Geometry: final body of the model. Coordinates: model frame, mm. A direction names the side the tool comes from. Round coordinates to 2 decimals unless told otherwise and drop trailing zeros. Order: outer loops, then holes, each group sorted by start corner. A loop starts at its lowest first (then second) coordinate and runs counter-clockwise, first axis right, second up. Notation, with made-up numbers: (85.5, 35.5) - (103.5, 35.5) arc R14 cw to (103.5, 61.5) - close; hole circle Ø6 at (30.25, 59). An arc over 180 degrees is marked (long way). Put each result on its own line as item: value. Start each with the question number.
(1) Section C-C (z = -8). Output: boundary loops of the cut face in (x, y).
(2) Pin query (flat end, axial travel): P1, Ø2, axis at x = 30.5, y = -4.5, coming from the -Z side; P2, Ø2, axis at x = -6.5, y = 57.5, coming from the -Z side; P3, Ø6, axis at x = 26.5, z = -12, coming from the -Y side. Return the tip coordinate at first contact, or that it passes through.
(3) Material intervals for L1, parallel to Y at x = -6.5, z = -17.75; L2, parallel to Y at x = -6.5, z = -13.75; L3, parallel to Y at x = 29.5, z = -10, sorted ascending. Write a range as [from, to].
(4) Access query for faces 4 (the face through (0.15, -11.25, 1.73)), 5 (the face through (0, 61, -16)), 6 (the face through (0, 55, -16)). Directions: +Z, -Z, +X, -X, +Y, -Y. A direction counts if a zero-diameter tool reaches every point of the face in a straight line with its end or side. Return the directions, or none.
(5) Section A-A (x = 0). Output: boundary loops of the cut face in (y, z).
(6) Pull-direction query (Z, two-part tool) for faces 1 (the face through (-0.15, 11.25, 1.73)), 2 (the face through (0, -55, -16)), 3 (the face through (10.892, 34.587, 1.745)); classes: released by +Z, released by -Z, zero draft, split by the parting line, or undercut.
(7) Section B-B (y = 0). Output: boundary loops of the cut face in (x, z), and give its area (3 significant figures).
Autodesk Inventor part; units mm, degrees
ref_plane "Work Plane2" through (0, 61, 0) normal (0, 1, 0) x (-1, 0, 0)
ref_plane "YZ Plane" through (0, 0, 0) normal (1, 0, 0) x (0, 1, 0)
ref_plane "XY Plane" through (0, 0, 0) normal (0, 0, 1) x (1, 0, 0)
sketch "Sketch1" plane through (0, 0, 0) normal (0, 0, 1) x (1, 0, 0)
  circle A0 centre (0, 0) radius 11.25
  line L0 (-9, 6.75) -> (-9, -6.75)
  line L1 (9, 6.75) -> (9, -6.75)
  circle A1 centre (0, 0) radius 32.5
  dimension "d0" = 22.5
  dimension "d1" = 18
  dimension "d2" = 65
extrude "Extrusion1" add sketch "Sketch1" along normal blind 3.5 contours A0 L1 | L0 A0 | A1
sketch "Sketch2" plane through (0, 0, 0) normal (1, 0, 0) x (0, 1, 0)
  line L0 (32.5, 0) -> (-32.5, 0)
  line L1 (32.5, 0) -> (55.5, -21.5)
  line L2 (55.5, -21.5) -> (62.5, -21.5)
  line L3 (62.5, -21.5) -> (62.5, -10.5)
  line L4 (32.5, 3.5) -> (-32.5, 3.5)
  line L5 (32.5, 3.5) -> (62.5, -10.5)
  line L6 (0, 0) -> (0, -19.375) construction
  line L7 (32.5, 3.5) -> (32.5, 0)
  dimension "d8" = 7
  dimension "d9" = 25
  dimension "d10" = 11
  dimension "d11" = 30
revolve "Revolution1" add sketch "Sketch2" angle 360 about axis through (0, 0, 0) along (0, 0, -1)
fillet "Fillet1" radius 10 1 edges at (0, -32.5, 3.5)
ref_plane "Work Plane2" through (0, 61, 0) normal (0, 1, 0) x (-1, 0, 0)
sketch "Sketch3" plane through (0, 61, 0) normal (0, 1, 0) x (-1, 0, 0)
  circle A0 centre (0, -16) radius 4.5
  line L0 (4.5, -16) -> (4.5, -20.5)
  line L1 (-4.5, -20.5) -> (-4.5, -16)
  line L2 (-62.5, -21.5) -> (62.5, -21.5)
  line L3 (62.5, -21.5) -> (62.5, -11.7) construction
  line L4 (62.5, -10.5) -> (62.5, -21.5)
  line L5 (-9, 0) -> (9, 0)
  line L6 (-4.5, -20.5) -> (4.5, -20.5)
  point P0 (0, 0)
  point P1 (0, 0)
  point P2 (0, -20.5)
  dimension "d14" = 9
  dimension "d22" = 1
extrude "Extrusion2" cut sketch "Sketch3" against normal blind 6
sketch "Sketch4" plane through (0, 0, 3.5) normal (0, 0, 1) x (1, 0, 0)
  circle A0 centre (0, 45) radius 9
  point P0 (0, 0)
  dimension "d25" = 45
  dimension "d26" = 18
extrude "Extrusion3" [suppressed]
pattern_circular "Circular Pattern1" [suppressed]
mirror "Mirror1" about plane through (0, 0, 0) normal (0, 1, 0) of "Extrusion2"
sketch "Sketch5" plane through (0, 0, -21.5) normal (0, 0, -1) x (-1, 0, 0)
  circle A0 centre (0, 0) radius 62.5
  circle A1 centre (0, 0) radius 55.5
extrude "Extrusion4" cut sketch "Sketch5" against normal blind 1
sketch "Sketch6" plane through (0, 0, -20.5) normal (0, 0, -1) x (-1, 0, 0)
  line L0 (-4.5, 61) -> (-4.5, 55)
  line L1 (-4.5, 58) -> (-6.5, 58)
  circle A0 centre (-6.5, 58) radius 1.25
  line L2 (0, 60.0655) -> (0, 54.4578) construction
  circle A1 centre (6.5, 58) radius 1.25
  circle A2 centre (0, 0) radius 55.5 construction
  line L3 (-55.5, 0) -> (55.5, 0) construction
  circle A3 centre (-6.5, -58) radius 1.25
  circle A4 centre (6.5, -58) radius 1.25
  dimension "d32" = 2
  dimension "d33" = 2.5
extrude "Extrusion5" cut sketch "Sketch6" against normal blind 10
properties part number "CVT_Ring"
Checks:
1. outline: circle Ø114.29 at (0, 0); hole circle Ø82.12 at (0, 0)
2. P1: stops at z = 0
2. P2: stops at z = -20.5
2. P3: stops at y = -57.91
3. L1: y = [-62.16, -59.25], [-56.75, -51.08], [51.08, 56.75], [59.25, 62.16]
3. L2: y = [-62.16, -59.25], [-56.75, -46.76], [46.76, 56.75], [59.25, 62.16]
3. L3: y = [-53.88, -31.56], [31.56, 53.88]
4. face 4: +Z, -Z
4. face 5: -Z
4. face 6: none
5. outline: (-62.5, -20.5) - (-61, -20.5) - (-61, -11.5) - (-55, -11.5) - (-55, -20.5) - (-55.5, -20.5) - (-55.5, -21.5) - (-32.5, 0) - (-11.25, 0) - (-11.25, 3.5) - (-30.28, 3.5) arc R10 ccw to (-34.51, 2.56) - (-62.5, -10.5) - close; (11.25, 0) - (32.5, 0) - (55.5, -21.5) - (55.5, -20.5) - (55, -20.5) - (55, -11.5) - (61, -11.5) - (61, -20.5) - (62.5, -20.5) - (62.5, -10.5) - (34.51, 2.56) arc R10 ccw to (30.28, 3.5) - (11.25, 3.5) - close
6. face 1: zero draft
6. face 2: undercut
6. face 3: released by +Z
7. outline: (-62.5, -20.5) - (-55.5, -20.5) - (-55.5, -21.5) - (-32.5, 0) - (-9, 0) - (-9, 3.5) - (-30.28, 3.5) arc R10 ccw to (-34.51, 2.56) - (-62.5, -10.5) - close; (9, 0) - (32.5, 0) - (55.5, -21.5) - (55.5, -20.5) - (62.5, -20.5) - (62.5, -10.5) - (34.51, 2.56) arc R10 ccw to (30.28, 3.5) - (9, 3.5) - close
7. area: 735 mm²
